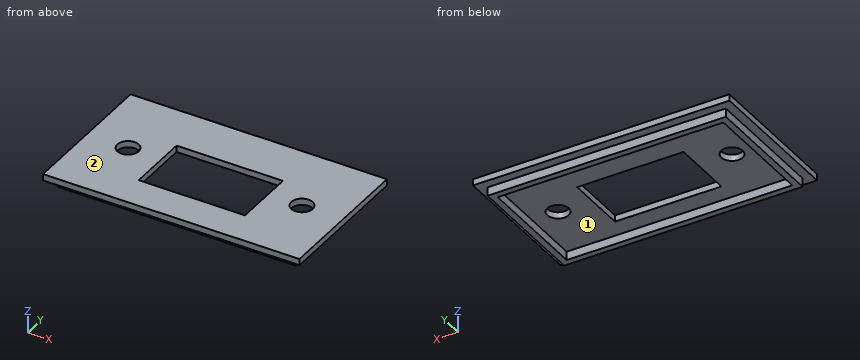
```python
from build123d import *

# Parameters (mm, degrees)
ESQUISSE2_W             = 55.8
ESQUISSE2_H             = 29.8
ESQUISSE2_W_2           = 52.8
ESQUISSE2_H_2           = 26.8
BOSS_EXTRU_1_DEPTH      = 2
ESQUISSE3_W             = 60
ESQUISSE3_H             = 34
BOSS_EXTRU_2_DEPTH      = 1.5
ESQUISSE4_W             = 24.9
ESQUISSE4_H             = 14.7
ENL_V_MAT_EXTRU_1_DEPTH = 1.5
ESQUISSE5_R             = 2.5
ENL_V_MAT_EXTRU_2_DEPTH = 1.5


with BuildPart() as part:
    # Esquisse2 → Boss.-Extru.1 (new body)
    with BuildSketch(Plane.XY):
        with Locations((0, 14.9)):
            Rectangle(ESQUISSE2_W, ESQUISSE2_H)
        with Locations((0, 14.9)):
            Rectangle(ESQUISSE2_W_2, ESQUISSE2_H_2, mode=Mode.SUBTRACT)
    extrude(amount=-BOSS_EXTRU_1_DEPTH)

    # Esquisse3 → Boss.-Extru.2 (add)
    with BuildSketch(Plane.XY):
        with Locations((0, 14.9)):
            Rectangle(ESQUISSE3_W, ESQUISSE3_H)
    extrude(amount=BOSS_EXTRU_2_DEPTH)

    # Esquisse4 → Enlèv. mat.-Extru.1 (cut)
    with BuildSketch(Plane.XY.offset(1.5)):
        with Locations((0, 13.25)):
            Rectangle(ESQUISSE4_W, ESQUISSE4_H)
    extrude(amount=-ENL_V_MAT_EXTRU_1_DEPTH, mode=Mode.SUBTRACT)

    # Esquisse5 → Enlèv. mat.-Extru.2 (cut)
    with BuildSketch(Plane(origin=(0, 0, 0), x_dir=(-1, 0, 0), z_dir=(0, 0, -1))):
        with Locations((20.35, 14.9)):
            Circle(ESQUISSE5_R)
        with Locations((-20.35, 14.9)):
            Circle(ESQUISSE5_R)
    extrude(amount=-ENL_V_MAT_EXTRU_2_DEPTH, mode=Mode.SUBTRACT)


solid = part.part
```
Here's how the part is built. I have some questions about the finished solid (model axes, mm). Face numbers are marked on the shaded views. Coordinates: 2 decimals unless noted, no trailing zeros. Write each loop counter-clockwise with the first axis right and the second up, starting at its lowest first coordinate (ties: lowest second). Pieces come first, ordered by that corner, then holes. Notation, with made-up numbers: (-8.5, 39) -> (39.5, 39) arc R13 cw to (39.5, 48) -> close; hole circle Ø9 at (1, 1). An arc over 180 degrees is marked (long way). Use a Markdown table: item, result. Add a question column.
(1) If we section it at B-B, the plane x = 20.35: Write out the boundary of the cut face in (y, z).
(2) If we section it at A-A, the plane y = 7: Write out the boundary of the cut face in (x, z), and give its area (4 significant figures).
(3) I'm going to push flat-ended pins straight in: P1, Ø2, axis at x = 10, z = -1.5, coming from the +Y side; P2, Ø13.5, axis at x = 10.5, y = 20.5, coming from the -Z side; P3, Ø1.6, axis at x = -2.5, z = -0.5, coming from the +Y side; P4, Ø4, axis at x = -20.35, y = 14.9, coming from the +Z side. Where does each tip first touch, or does it pass through?
(4) We'd pull the mould along X, two halves only. Please class the marked faces 1 and 2: +X half, -X half, draft (parallel to the pull), parting line (faces both ways), or undercut.
(5) If we section it at D-D, the plane y = 14.9: Write out the boundary of the cut face in (x, z), and give its area (4 significant figures).
(6) Please list where these lines run through material, in increasing order: line 1 (Y direction, x = 16.5, z = -0.95); line 2 (Y direction, x = 20.35, z = 0.85); line 3 (X direction, y = 14.5, z = -1.6).
(7) If we section it at C-C, the plane z = -1.3: Write out the boundary of the cut face in (x, y).
Outcome:
| question | item | result |
|---|---|---|
| 1 | outline | (-2.1, 0) -> (0, 0) -> (0, -2) -> (1.5, -2) -> (1.5, 0) -> (12.4, 0) -> (12.4, 1.5) -> (-2.1, 1.5) -> close; (17.4, 0) -> (28.3, 0) -> (28.3, -2) -> (29.8, -2) -> (29.8, 0) -> (31.9, 0) -> (31.9, 1.5) -> (17.4, 1.5) -> close |
| 2 | outline | (-30, 0) -> (-27.9, 0) -> (-27.9, -2) -> (-26.4, -2) -> (-26.4, 0) -> (-12.45, 0) -> (-12.45, 1.5) -> (-30, 1.5) -> close; (12.45, 0) -> (26.4, 0) -> (26.4, -2) -> (27.9, -2) -> (27.9, 0) -> (30, 0) -> (30, 1.5) -> (12.45, 1.5) -> close |
| 2 | area | 58.65 mm^2 |
| 3 | P1 | stops at y = 29.8 |
| 3 | P2 | stops at z = 0 |
| 3 | P3 | stops at y = 31.9 |
| 3 | P4 | passes through |
| 4 | face 1 | undercut |
| 4 | face 2 | draft |
| 5 | outline | (-30, 0) -> (-27.9, 0) -> (-27.9, -2) -> (-26.4, -2) -> (-26.4, 0) -> (-22.85, 0) -> (-22.85, 1.5) -> (-30, 1.5) -> close; (-17.85, 0) -> (-12.45, 0) -> (-12.45, 1.5) -> (-17.85, 1.5) -> close; (12.45, 0) -> (17.85, 0) -> (17.85, 1.5) -> (12.45, 1.5) -> close; (22.85, 0) -> (26.4, 0) -> (26.4, -2) -> (27.9, -2) -> (27.9, 0) -> (30, 0) -> (30, 1.5) -> (22.85, 1.5) -> close |
| 5 | area | 43.65 mm^2 |
| 6 | line 1 | y = 0 to 1.5, 28.3 to 29.8 |
| 6 | line 2 | y = -2.1 to 12.4, 17.4 to 31.9 |
| 6 | line 3 | x = -27.9 to -26.4, 26.4 to 27.9 |
| 7 | outline | (-27.9, 0) -> (27.9, 0) -> (27.9, 29.8) -> (-27.9, 29.8) -> close; hole (-26.4, 1.5) -> (26.4, 1.5) -> (26.4, 28.3) -> (-26.4, 28.3) -> close |
